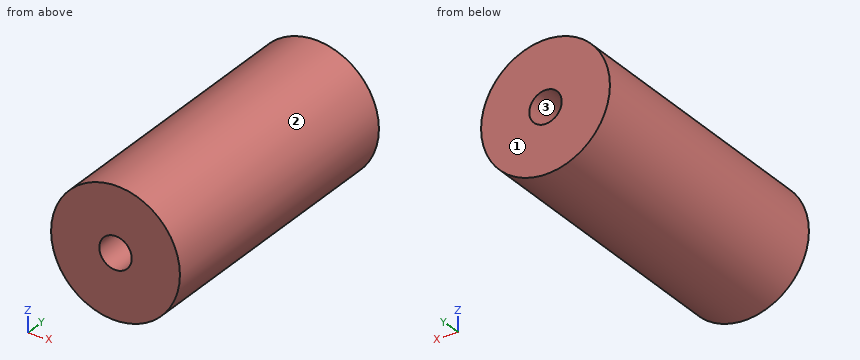
Autodesk Inventor part; units mm, degrees
ref_plane "YZ Plane" through (0, 0, 0) normal (1, 0, 0) x (0, 1, 0)
ref_plane "XZ Plane" through (0, 0, 0) normal (0, 1, 0) x (-1, 0, 0)
ref_plane "XY Plane" through (0, 0, 0) normal (0, 0, 1) x (1, 0, 0)
sketch "Boceto1" plane through (0, 0, 0) normal (0, 1, 0) x (-1, 0, 0)
  circle A0 centre (0, 0) radius 9.9365
extrude "Extrusión1" add sketch "Boceto1" along normal blind 30
extrude "Extrusión2" cut sketch "Boceto1" along normal blind 30
extrude "Extrusión3" add sketch "Boceto1" along normal blind 45
sketch "Boceto2" plane through (0, 45, 0) normal (0, 1, 0) x (1, 0, 0)
  point P0 (0, 0)
hole "Agujero1" at (0, 45, 0) direction (0, -1, 0) diameter 5 end through all
properties part number "pieza base de bobina"
Here's how the part is built. I have some questions about the finished solid (model axes, mm). Face numbers are marked on the shaded views. Give positions to 0.01 mm unless a question says otherwise; leave off trailing zeros. Write each loop counter-clockwise with the first axis right and the second up, starting at its lowest first coordinate (ties: lowest second). Pieces come first, ordered by that corner, then holes.
(1) Will these pins go through, and if not, where does the flat tip stop? pin 1 (2 mm diameter, centred on x = 3, y = 27, fed in from -Z); pin 2 (3 mm diameter, centred on y = 7, z = 2, fed in from +X); pin 3 (4.5 mm diameter, centred on x = 0, z = 0, fed in from +Y); pin 4 (1 mm diameter, centred on x = -6.5, y = 32.5, fed in from -Z).
Output values:
pin 1: stops at z = -9.73
pin 2: stops at x = 9.92
pin 3: passes through
pin 4: stops at z = -7.92
(2) Imagine slicing it at B-B, the plane x = 0. Write out the boundary of the cut face in (y, z), and give its area (3 significant figures).
Output values:
outline: (0, -9.94) - (45, -9.94) - (45, -2.5) - (0, -2.5) - close; (0, 2.5) - (45, 2.5) - (45, 9.94) - (0, 9.94) - close
area: 669 mm2
(3) Imagine slicing it at C-C, the plane y = 28.5. Write out the boundary of the cut face in (x, z), and give its area (3 significant figures).
Output values:
outline: circle Ø19.87 at (0, 0); hole circle Ø5 at (0, 0)
area: 291 mm2
(4) Imagine slicing it at D-D, the plane x = -4.25. Write out the boundary of the cut face in (y, z).
Output values:
outline: (0, -8.98) - (45, -8.98) - (45, 8.98) - (0, 8.98) - close
(5) Imagine slicing it at A-A, the plane z = 0. Write out the boundary of the cut face in (x, y).
Output values:
outline: (-9.94, 0) - (-2.5, 0) - (-2.5, 45) - (-9.94, 45) - close; (2.5, 0) - (9.94, 0) - (9.94, 45) - (2.5, 45) - close
(6) If I drill on L1, parallel to Z at x = 0, y = 25; L2, parallel to X at y = 5, z = 0.25; L3, parallel to X at y = 41, z = 6.5, over which ranges is the centre line in solid material (lowest first)?
Output values:
L1: z = -9.94 to -2.5, 2.5 to 9.94
L2: x = -9.93 to -2.49, 2.49 to 9.93
L3: x = -7.52 to 7.52
(7) Thinking about a two-plate mould opening in X: for the marked faces 1, 2 and 3, which applies, pulls with the +X half, pulls with the -X half, needs draft (parallel to the pull), parting line crosses it, or undercut?
Output values:
face 1: needs draft
face 2: parting line crosses it
face 3: undercut
